Input: part model. Units: mm. Frame: model coordinates. Face numbers are marked on the shaded views. A direction names the side the tool comes from. Round coordinates to 2 decimals unless told otherwise and drop trailing zeros. Loops run counter-clockwise (first coordinate to the right, second up) from the corner with the lowest first, then second, coordinate; pieces in that order, holes last. Notation, with made-up numbers: (42, -26.75) -> (99, -26.75) arc R24 cw to (99, -9.75) -> close; hole circle Ø5 at (58, 57.5). An arc over 180 degrees is marked (long way). Answer as a JSON object with one key per item and string values.
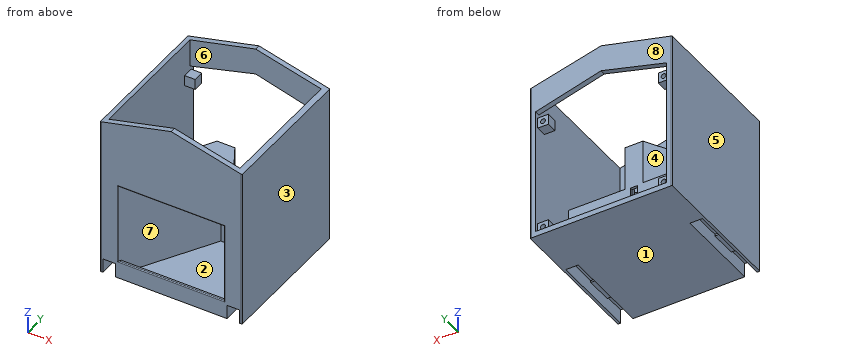
```python
from build123d import *

# Parameters (mm, degrees)
PAD_DEPTH       = 160
SKETCH001_W     = 120
SKETCH001_H     = 90
POCKET_DEPTH    = 100
PAD001_DEPTH    = 90
POCKET001_DEPTH = 16
POCKET002_DEPTH = 60
SKETCH006_W     = 148
SKETCH006_H     = 148
POCKET004_DEPTH = 80
SKETCH007_W     = 14
SKETCH007_H     = 16
SKETCH007_W_2   = 14.0000000001
SKETCH007_H_2   = 15.9999999999
POCKET005_DEPTH = 100
SKETCH008_W     = 14
SKETCH008_H     = 30
SKETCH008_W_2   = 14.0000000001
SKETCH008_H_2   = 29.9999999999
PAD002_DEPTH    = 2
POCKET008_DEPTH = 10
POCKET009_DEPTH = 50
SKETCH009_R     = 2.5
POCKET010_DEPTH = 10
SKETCH005_W     = 8
SKETCH005_H     = 16
POCKET011_DEPTH = 5
SKETCH012_R     = 6
POCKET012_DEPTH = 10
SKETCH013_R     = 2.75
POCKET013_DEPTH = 5
SKETCH015_R     = 6
POCKET014_DEPTH = 10
SKETCH016_R     = 2.75
POCKET015_DEPTH = 5
SKETCH017_W     = 12
SKETCH017_H     = 12
PAD003_DEPTH    = 12
SKETCH018_W     = 12
SKETCH018_H     = 12
PAD004_DEPTH    = 12
SKETCH019_R     = 2.75
POCKET016_DEPTH = 9
FILLET_R        = 1


with BuildPart() as part:
    # Sketch → Pad (new body)
    with BuildSketch(Plane.XZ):
        Polygon((0, 0), (0, 180), (80, 200), (160, 180), (160, 0), align=None)
    extrude(amount=-PAD_DEPTH)

    # Sketch001 (on Face6 of Pad) → Pocket (cut)
    with BuildSketch(Plane.XZ):
        with Locations((80, 65)):
            Rectangle(SKETCH001_W, SKETCH001_H)
    extrude(amount=-POCKET_DEPTH, mode=Mode.SUBTRACT)

    # Sketch002 (on Face10 of Pocket) → Pad001 (join)
    with BuildSketch(Plane(origin=(0, 0, 20), x_dir=(-1, 0, 0), z_dir=(0, 0, 1))):
        Polygon((-20, 0), (-76, -96.9948452239), (-84, -96.9948452239), (-140, 0), (-140, -100), (-20, -100), align=None)
    extrude(amount=PAD001_DEPTH)

    # Sketch003 (on Face10 of Pad001) → Pocket001 (cut)
    with BuildSketch(Plane(origin=(0, 0, 20), x_dir=(-1, 0, 0), z_dir=(0, 0, 1))):
        Polygon((-21.7320508076, -3), (-138.2679491924, -3), (-84, -96.9948452239), (-76, -96.9948452239), align=None)
    extrude(amount=-POCKET001_DEPTH, mode=Mode.SUBTRACT)

    # Sketch004 (on Face5 of Pocket001) → Pocket002 (cut)
    with BuildSketch(Plane(origin=(0, 160, 0), x_dir=(1, 0, 0), z_dir=(0, 1, 0))):
        Polygon((6, -150), (6, -6), (154, -6), (154, -150), (80, -170), align=None)
    extrude(amount=-POCKET002_DEPTH, mode=Mode.SUBTRACT)

    # Sketch006 → Pocket004 (cut)
    with BuildSketch(Plane.XY.offset(200)):
        with Locations((80, 80)):
            Rectangle(SKETCH006_W, SKETCH006_H)
    extrude(amount=-POCKET004_DEPTH, mode=Mode.SUBTRACT)

    # Sketch007 (on Face4 of Pocket004) → Pocket005 (cut)
    with BuildSketch(Plane.XZ):
        with Locations((10, 8)):
            Rectangle(SKETCH007_W, SKETCH007_H)
        with Locations((150, 8)):
            Rectangle(SKETCH007_W_2, SKETCH007_H_2)
    extrude(amount=-POCKET005_DEPTH, mode=Mode.SUBTRACT)

    # Sketch008 (on Face17 of Pocket005) → Pad002 (join)
    with BuildSketch(Plane(origin=(0, 0, 16), x_dir=(1, 0, 0), z_dir=(0, 0, -1))):
        with Locations((10, -39.5)):
            Rectangle(SKETCH008_W, SKETCH008_H)
        with Locations((150, -39.5)):
            Rectangle(SKETCH008_W_2, SKETCH008_H_2)
    extrude(amount=PAD002_DEPTH)

    # Sketch010 → Pocket008 (cut)
    with BuildSketch(Plane(origin=(0, 0, 110), x_dir=(1, 0, 0), z_dir=(0, 0, -1))):
        Polygon((40, -34.6410161514), (60, -69.2820323028), (72.9903810568, -61.7820323028), (52.9903810568, -27.1410161514), align=None)
        Polygon((107.0096189432, -27.1410161514), (87.0096189432, -61.7820323028), (100, -69.2820323028), (120, -34.6410161514), align=None)
    extrude(amount=-POCKET008_DEPTH, mode=Mode.SUBTRACT)

    # Sketch011 (on Face39 of Pocket008) → Pocket009 (cut)
    with BuildSketch(Plane(origin=(0, 0, 120), x_dir=(-1, 0, 0), z_dir=(0, 0, 1))):
        Polygon((-130.4145188433, -30), (-90, -100), (-154, -100), (-154, -30), align=None)
        Polygon((-29.5854811567, -30), (-70, -100), (-6, -100), (-6, -30), align=None)
    extrude(amount=-POCKET009_DEPTH, mode=Mode.SUBTRACT)

    # Sketch009 (on Face29 of Pocket009) → Pocket010 (cut)
    with BuildSketch(Plane(origin=(0, 0, 14), x_dir=(1, 0, 0), z_dir=(0, 0, -1))):
        with Locations((10, -34.5)):
            Circle(SKETCH009_R)
        with Locations((10, -44.5)):
            Circle(SKETCH009_R)
        with Locations((150, -34.5)):
            Circle(SKETCH009_R)
        with Locations((150, -44.5)):
            Circle(SKETCH009_R)
    extrude(amount=-POCKET010_DEPTH, mode=Mode.SUBTRACT)

    # Sketch005 (on Face44 of Pocket009) → Pocket011 (cut)
    with BuildSketch(Plane.XZ.offset(-96.9948452239)):
        with Locations((80, 61)):
            Rectangle(SKETCH005_W, SKETCH005_H)
    extrude(amount=-POCKET011_DEPTH, mode=Mode.SUBTRACT)

    # Sketch012 (on Face61 of Pocket011) → Pocket012 (cut)
    with BuildSketch(Plane(origin=(9.1987298108, -5.3108891325, 0), x_dir=(0, 0, -1), z_dir=(-0.8660254038, 0.5, 0))):
        with Locations((-115, -70)):
            Circle(SKETCH012_R)
    extrude(amount=-POCKET012_DEPTH, mode=Mode.SUBTRACT)

    # Sketch013 (on Face64 of Pocket012) → Pocket013 (cut)
    with BuildSketch(Plane(origin=(9.1987298108, -5.3108891325, 0), x_dir=(0, 0, -1), z_dir=(-0.8660254038, 0.5, 0))):
        with Locations((-107, -52.5)):
            Circle(SKETCH013_R)
        with Locations((-107, -87.5)):
            Circle(SKETCH013_R)
    extrude(amount=-POCKET013_DEPTH, mode=Mode.SUBTRACT)

    # Sketch015 (on Face65 of Pocket013) → Pocket014 (cut)
    with BuildSketch(Plane(origin=(110.8012701892, 63.9711431703, 0), x_dir=(0, 0, 1), z_dir=(0.8660254038, 0.5, 0))):
        with Locations((115, 10)):
            Circle(SKETCH015_R)
    extrude(amount=-POCKET014_DEPTH, mode=Mode.SUBTRACT)

    # Sketch016 (on Face67 of Pocket014) → Pocket015 (cut)
    with BuildSketch(Plane(origin=(110.8012701892, 63.9711431703, 0), x_dir=(0, 0, 1), z_dir=(0.8660254038, 0.5, 0))):
        with Locations((107, 27.5)):
            Circle(SKETCH016_R)
        with Locations((107, -7.5)):
            Circle(SKETCH016_R)
    extrude(amount=-POCKET015_DEPTH, mode=Mode.SUBTRACT)

    # Sketch017 (on Face25 of Pocket015) → Pad003 (join)
    with BuildSketch(Plane(origin=(154, 0, 0), x_dir=(0, 0, -1), z_dir=(-1, 0, 0))):
        with Locations((-12, -150)):
            Rectangle(SKETCH017_W, SKETCH017_H)
        with Locations((-139, -150)):
            Rectangle(SKETCH017_W, SKETCH017_H)
    extrude(amount=PAD003_DEPTH)

    # Sketch018 (on Face27 of Pad003) → Pad004 (join)
    with BuildSketch(Plane(origin=(6, 0, 0), x_dir=(0, 0, 1), z_dir=(1, 0, 0))):
        with Locations((12, -150)):
            Rectangle(SKETCH018_W, SKETCH018_H)
        with Locations((139, -150)):
            Rectangle(SKETCH018_W, SKETCH018_H)
    extrude(amount=PAD004_DEPTH)

    # Sketch019 (on Face68 of Pad004) → Pocket016 (cut)
    with BuildSketch(Plane(origin=(0, 156, 0), x_dir=(1, 0, 0), z_dir=(0, 1, 0))):
        with Locations((148, -12)):
            Circle(SKETCH019_R)
        with Locations((148, -139)):
            Circle(SKETCH019_R)
        with Locations((12, -139)):
            Circle(SKETCH019_R)
        with Locations((12, -12)):
            Circle(SKETCH019_R)
    extrude(amount=-POCKET016_DEPTH, mode=Mode.SUBTRACT)

    # Fillet
    fillet_edges = [part.edges().sort_by_distance(p)[0] for p in [
        (0, 160, 90),
        (0, 0, 90),
        (160, 0, 90),
        (80, 0, 20),
        (20, 0, 65),
        (80, 0, 110),
        (140, 0, 65),
        (160, 160, 90),
    ]]
    fillet(fillet_edges, radius=FILLET_R)


solid = part.part
```
1) Ray query, probe 1 along Z at (x, y) = (12, 151.5); probe 2 along X at (y, z) = (149.75, 139); probe 3 along X at (y, z) = (74, 140). Return the intervals inside material, ascending.
Output:
{"probe 1": "z = 0 to 9.25, 14.75 to 18, 133 to 136.25, 141.75 to 145", "probe 2": "x = 0 to 9.25, 14.75 to 18, 142 to 145.25, 150.75 to 160", "probe 3": "x = 0 to 6, 154 to 160"}
2) Section B-B, the plane z = 139. Output: boundary loops of the cut face in (x, y).
Output:
{"outline": "(0, 1) arc R1 ccw to (1, 0) -> (159, 0) arc R1 ccw to (160, 1) -> (160, 159) arc R1 ccw to (159, 160) -> (154, 160) -> (154, 156) -> (150.75, 156) -> (150.75, 147) -> (145.25, 147) -> (145.25, 156) -> (142, 156) -> (142, 144) -> (154, 144) -> (154, 6) -> (6, 6) -> (6, 144) -> (18, 144) -> (18, 156) -> (14.75, 156) -> (14.75, 147) -> (9.25, 147) -> (9.25, 156) -> (6, 156) -> (6, 160) -> (1, 160) arc R1 ccw to (0, 159) -> close"}
3) Draft query along Z for the marked faces 1, 2 and 3. Return one class per face: +Z half, -Z half, draft (parallel to the pull), parting line (faces both ways), or undercut.
Output:
{"face 1": "-Z half", "face 2": "undercut", "face 3": "draft"}
4) Contact query for flat-ended pins moving along their axis: P1, Ø4, axis at x = 93, y = 133, coming from the +Z side; P2, Ø1.5, axis at x = 25.5, z = 45, coming from the -Y side; P3, Ø1.5, axis at x = 150.5, y = 43.5, coming from the -Z side. Output: stop coordinate, or through.
Output:
{"P1": "stops at z = 6", "P2": "stops at y = 8.23", "P3": "stops at z = 24"}
5) Section A-A, the plane y = 130. Output: boundary loops of the cut face in (x, z).
Output:
{"outline": "(0, 0) -> (160, 0) -> (160, 180) -> (154, 181.5) -> (154, 6) -> (6, 6) -> (6, 181.5) -> (0, 180) -> close"}
6) Reachability of the marked faces 4, 5, 6, 7 and 8 from +Z, -Z, +X, -X, +Y, -Y: full face, straight path, thin tool, end or side. Return the list, or none.
Output:
{"face 4": "+Z, +Y", "face 5": "+Z, -Z, -X, +Y, -Y", "face 6": "+Z", "face 7": "none", "face 8": "+Z, -Z, +X, -X, +Y"}
7) Section C-C, the plane z = 27. Output: boundary loops of the cut face in (x, y).
Output:
{"outline": "(0, 1) arc R1 ccw to (1, 0) -> (19.42, 0) arc R1 ccw to (20.29, 0.5) -> (76, 96.99) -> (84, 96.99) -> (139.71, 0.5) arc R1 ccw to (140.58, 0) -> (159, 0) arc R1 ccw to (160, 1) -> (160, 159) arc R1 ccw to (159, 160) -> (154, 160) -> (154, 100) -> (6, 100) -> (6, 160) -> (1, 160) arc R1 ccw to (0, 159) -> close"}
